Source: CAD feature listing. Evaluate the final solid. Frame: model axes, mm. Round coordinates to 2 decimals unless told otherwise and drop trailing zeros. Order: outer loops, then holes, each group sorted by start corner. A loop starts at its lowest first (then second) coordinate and runs counter-clockwise, first axis right, second up. Notation, with made-up numbers: (30.25, 62) - (37.25, 62) arc R16 ccw to (37.25, 75) - close; hole circle Ø10 at (1.5, 13.25). An arc over 180 degrees is marked (long way). Use one line per item in the form item = value. Start each with the question number.
Q1. Cut plane D-D, the plane y = 3.4. Give the number of separate pieces and of enclosed holes in the cut face, and give its area (3 significant figures).
Q2. Cut plane A-A, the plane x = -9. Return the cut outline in (y, z).
Q3. Cut plane B-B, the plane x = -23.57. Return the cut outline in (y, z).
Q4. Ray query, line 1 (X direction, y = 2.35, z = 17); line 2 (Z direction, x = 15, y = 3.5); line 3 (X direction, y = 0.7, z = -16.5). Return the intervals inside material, ascending. Write a range as [from, to].
Q5. Cut plane C-C, the plane z = 7.5. Return the cut outline in (x, y), and give its area (3 significant figures).
Q6. Pin query (flat end, axial travel): pin 1 Ø2 at (y, z) = (2.5, -15) entering from +X; pin 2 Ø4 at (x, z) = (-15.56, 15.56) entering from -Y; pin 3 Ø1.5 at (x, y) = (6, 0.5) entering from -Z. Return the tip coordinate at first contact, or that it passes through.
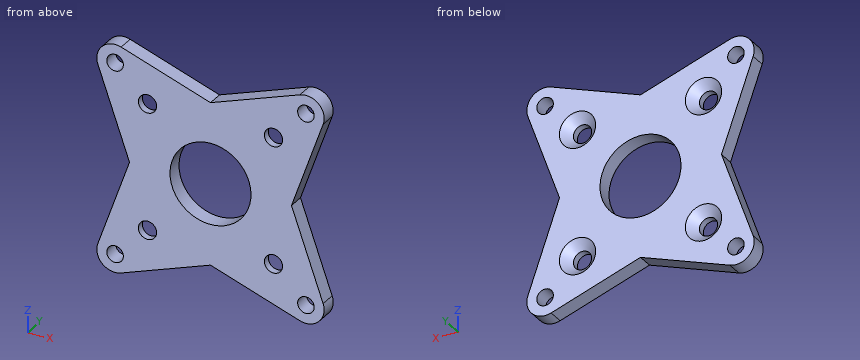
from build123d import *

# Parameters (mm, degrees)
SKETCH1_W                                    = 71.3
SKETCH1_H                                    = 60
BOSS_EXTRUDE1_DEPTH                          = 4
SKETCH2_R                                    = 2.05
CUT_EXTRUDE1_DEPTH                           = 47.764543192
SKETCH4_R                                    = 10
CUT_EXTRUDE3_DEPTH                           = 47.764543192
SKETCH5_OUTSIDE_W                            = 91.954
SKETCH5_OUTSIDE_H                            = 80.654
CUT_EXTRUDE4_DEPTH                           = 47.764543192
CSK_FOR_M4_HEX_SOCKET_COUNTERSUNK_CA_2_COUNT = 2
CSK_FOR_M4_HEX_SOCKET_COUNTERSUNK_CA_2_PITCH = 31.112698372
CSK_FOR_M4_HEX_SOCKET_COUNTERSUNK_CA_3_COUNT = 2
CSK_FOR_M4_HEX_SOCKET_COUNTERSUNK_CA_3_PITCH = 44
CSK_FOR_M4_HEX_SOCKET_COUNTERSUNK_CA_4_COUNT = 2
CSK_FOR_M4_HEX_SOCKET_COUNTERSUNK_CA_4_PITCH = 31.112698372


with BuildPart() as part:
    # Sketch1 → Boss-Extrude1 (new body)
    with BuildSketch(Plane(origin=(0, 0, 0), x_dir=(1, 0, 0), z_dir=(0, 1, 0))):
        Rectangle(SKETCH1_W, SKETCH1_H)
    extrude(amount=BOSS_EXTRUDE1_DEPTH)

    # Sketch2 → Cut-Extrude1 (cut, through all)
    with BuildSketch(Plane(origin=(0, 4, 0), x_dir=(1, 0, 0), z_dir=(0, 1, 0))):
        with Locations(Location((-15.556349186, 15.556349186, 0), (0, 0, 270))):
            Circle(SKETCH2_R)
        with Locations(Location((-23.57, 23.57, 0), (0, 0, 270))):
            Circle(SKETCH2_R)
        with Locations(Location((15.556349186, 15.556349186, 0), (0, 0, 270))):
            Circle(SKETCH2_R)
        with Locations(Location((23.57, 23.57, 0), (0, 0, 270))):
            Circle(SKETCH2_R)
        with Locations(Location((15.556349186, -15.556349186, 0), (0, 0, 270))):
            Circle(SKETCH2_R)
        with Locations(Location((23.57, -23.57, 0), (0, 0, 270))):
            Circle(SKETCH2_R)
        with Locations(Location((-15.556349186, -15.556349186, 0), (0, 0, 270))):
            Circle(SKETCH2_R)
        with Locations(Location((-23.57, -23.57, 0), (0, 0, 270))):
            Circle(SKETCH2_R)
    extrude(amount=-CUT_EXTRUDE1_DEPTH, mode=Mode.SUBTRACT)

    # Sketch4 → Cut-Extrude3 (cut, through all)
    with BuildSketch(Plane(origin=(0, 4, 0), x_dir=(1, 0, 0), z_dir=(0, 1, 0))):
        with Locations(Location((0, 0, 0), (0, 0, 270))):
            Circle(SKETCH4_R)
    extrude(amount=-CUT_EXTRUDE3_DEPTH, mode=Mode.SUBTRACT)

    # Sketch5 outside → Cut-Extrude4 (cut, through all)
    with BuildSketch(Plane(origin=(0, 4, 0), x_dir=(1, 0, 0), z_dir=(0, 1, 0))):
        Rectangle(SKETCH5_OUTSIDE_W, SKETCH5_OUTSIDE_H)
        with BuildLine():
            Line((20, 0), (27.812053359, 22.068339818))
            ThreePointArc((27.812053359, 22.068339818), (26.751980515, 26.751980515), (22.068339818, 27.812053359))
            Line((22.068339818, 27.812053359), (0, 20))
            Line((0, 20), (-22.068339818, 27.812053359))
            ThreePointArc((-22.068339818, 27.812053359), (-26.751980515, 26.751980515), (-27.812053359, 22.068339818))
            Line((-27.812053359, 22.068339818), (-20, 0))
            Line((-20, 0), (-27.812053359, -22.068339818))
            ThreePointArc((-27.812053359, -22.068339818), (-26.751980515, -26.751980515), (-22.068339818, -27.812053359))
            Line((-22.068339818, -27.812053359), (0, -20))
            Line((0, -20), (22.068339818, -27.812053359))
            ThreePointArc((22.068339818, -27.812053359), (26.751980515, -26.751980515), (27.812053359, -22.068339818))
            Line((27.812053359, -22.068339818), (20, 0))
        make_face(mode=Mode.SUBTRACT)
    extrude(amount=-CUT_EXTRUDE4_DEPTH, mode=Mode.SUBTRACT)

    # Sketch7 → CSK for M4 Hex Socket Countersunk Cap Screw1 (revolve, cut)
    with BuildSketch(Plane(origin=(-15.556349186, 4, -15.556349186), x_dir=(0, 0, 1), z_dir=(1, 0, 0))):
        Polygon((0, 0), (0, 4), (2.25, 4), (2.25, 2.23), (4.48, 0), align=None)
    csk_for_m4_hex_socket_countersunk_cap_sc = revolve(axis=Axis((-15.556349186, 10.35, -15.556349186), (0, -1, 0)), mode=Mode.SUBTRACT)

    # CSK for M4 Hex Socket Countersunk Ca 2: CSK for M4 Hex Socket Countersunk Cap Screw1 ×2
    with Locations(*[(i * CSK_FOR_M4_HEX_SOCKET_COUNTERSUNK_CA_2_PITCH, 0, 0) for i in range(1, CSK_FOR_M4_HEX_SOCKET_COUNTERSUNK_CA_2_COUNT)]):
        add(csk_for_m4_hex_socket_countersunk_cap_sc, mode=Mode.SUBTRACT)

    # CSK for M4 Hex Socket Countersunk Ca 3: CSK for M4 Hex Socket Countersunk Cap Screw1 ×2
    with Locations(*[Vector(0.7071067811865476, 0, 0.7071067811865476) * (i * CSK_FOR_M4_HEX_SOCKET_COUNTERSUNK_CA_3_PITCH) for i in range(1, CSK_FOR_M4_HEX_SOCKET_COUNTERSUNK_CA_3_COUNT)]):
        add(csk_for_m4_hex_socket_countersunk_cap_sc, mode=Mode.SUBTRACT)

    # CSK for M4 Hex Socket Countersunk Ca 4: CSK for M4 Hex Socket Countersunk Cap Screw1 ×2
    with Locations(*[(0, 0, i * CSK_FOR_M4_HEX_SOCKET_COUNTERSUNK_CA_4_PITCH) for i in range(1, CSK_FOR_M4_HEX_SOCKET_COUNTERSUNK_CA_4_COUNT)]):
        add(csk_for_m4_hex_socket_countersunk_cap_sc, mode=Mode.SUBTRACT)


solid = part.part
Completed:
q1.separate_pieces = 1
q1.enclosed_holes = 9
q1.area = 1,840 mm2
q2.outline = (0, -23.19) - (4, -23.19) - (4, -4.36) - (0, -4.36) - close; (0, 4.36) - (4, 4.36) - (4, 23.19) - (0, 23.19) - close
q3.outline = (0, -28.07) - (4, -28.07) - (4, -25.62) - (0, -25.62) - close; (0, -21.52) - (4, -21.52) - (4, -10.08) - (0, -10.08) - close; (0, 10.08) - (4, 10.08) - (4, 21.52) - (0, 21.52) - close; (0, 25.62) - (4, 25.62) - (4, 28.07) - (0, 28.07) - close
q4.line_1 = [-26.02, -17.99], [-13.12, 13.12], [17.99, 26.02]
q4.line_2 = [-25.31, -19.5], [-11.62, 11.62], [19.5, 25.31]
q4.line_3 = [-25.84, -17.6], [-13.51, 13.51], [17.6, 25.84]
q5.outline = (-22.65, 0) - (-6.61, 0) - (-6.61, 4) - (-22.65, 4) - close; (6.61, 0) - (22.65, 0) - (22.65, 4) - (6.61, 4) - close
q5.area = 128 mm2
q6.pin_1 = 25.66
q6.pin_2 = through
q6.pin_3 = -22.39
